Could you check a few things on this model? Use its own coordinates, in mm. A direction names the side the tool comes from. Give positions to 0.01 mm unless a question says otherwise; leave off trailing zeros. Write each loop counter-clockwise with the first axis right and the second up, starting at its lowest first coordinate (ties: lowest second). Pieces come first, ordered by that corner, then holes. Notation, with made-up numbers: M -2,-12 L 45,-12 A22 ccw 45,22 Z; hole C 56.5,81 d1. An arc over 180 degrees is marked long. One line per item, written item: value.
```python
from build123d import *

# Parameters (mm, degrees)
CYLINDER040_R     = 2.5
CYLINDER040_DEPTH = 20
CYLINDER039_R     = 2.5
CYLINDER039_DEPTH = 20
BOX012_W          = 10
BOX012_H          = 12
BOX012_DEPTH      = 120
BOX013_W          = 20
BOX013_H          = 40
BOX013_DEPTH      = 120


with BuildPart() as cilindro027:
    # Cylinder040 → Cylinder040 (new body)
    with BuildSketch(Plane(origin=(-10, 59, 115), x_dir=(0, 0, -1), z_dir=(1, 0, 0))):
        Circle(CYLINDER040_R)
    extrude(amount=CYLINDER040_DEPTH)


with BuildPart() as obj1:
    # Cylinder039 → Cylinder039 (new body)
    with BuildSketch(Plane(origin=(-10, 59, 5), x_dir=(0, 0, -1), z_dir=(1, 0, 0))):
        Circle(CYLINDER039_R)
    extrude(amount=CYLINDER039_DEPTH)

    # Fusion021: union Cilindro027
    add(cilindro027.part)


with BuildPart() as obj1_1:
    # Fusion021 placement: moved
    add(obj1.part.moved(Location((0, -60, 0))))


with BuildPart() as cubo012:
    # Box012 → Box012 (new body)
    with BuildSketch(Plane(origin=(-5, -72, 0), x_dir=(1, 0, 0), z_dir=(0, 0, 1))):
        with Locations((5, 6)):
            Rectangle(BOX012_W, BOX012_H)
    extrude(amount=BOX012_DEPTH)


with BuildPart() as cut037:
    # Box013 → Box013 (new body)
    with BuildSketch(Plane(origin=(-10, -100, 0), x_dir=(1, 0, 0), z_dir=(0, 0, 1))):
        with Locations((10, 20)):
            Rectangle(BOX013_W, BOX013_H)
    extrude(amount=BOX013_DEPTH)

    # Cut036: cut Cubo012
    add(cubo012.part, mode=Mode.SUBTRACT)


with BuildPart() as cut037_1:
    # Cut036 placement: moved
    add(cut037.part.moved(Location((0, 64, 0))))

    # Cut037: cut obj1
    add(obj1_1.part, mode=Mode.SUBTRACT)


solid = cut037_1.part
```
1) If we section it at C-C, the plane z = 101: Write out the boundary of the cut face in (x, y).
Outcome:
outline: M -10,-36 L 10,-36 L 10,4 L 5,4 L 5,-8 L -5,-8 L -5,4 L -10,4 Z
2) Please list where these lines run through material, in increasing order: L1, parallel to Z at x = 8.55, y = -1; L2, parallel to Y at x = 7.45, z = 115; L3, parallel to X at y = -4, z = 80. Write a range as from..to.
Outcome:
L1: z = 0..2.5, 7.5..112.5, 117.5..120
L2: y = -36..-3.5, 1.5..4
L3: x = -10..-5, 5..10
3) If we section it at D-D, the plane x = -3: Write out the boundary of the cut face in (y, z).
Outcome:
outline: M -36,0 L -8,0 L -8,120 L -36,120 Z
4) On a 3-axis mill with a long thin cutter (end or side, diameter ignored), from which of +Z, -Z, +X, -X, +Y, -Y can I reach the whole of each face in a straight line? I mean faces 1 (the face through (-7.535, -0.249, 2.615)), 2 (the face through (-5, -2, 59)). Say none if no direction works.
Outcome:
face 1: +X, -X
face 2: +Z, -Z, +Y
5) If we section it at A-A, the plane z = 115: Write out the boundary of the cut face in (x, y).
Outcome:
outline: M -10,-36 L 10,-36 L 10,-3.5 L 5,-3.5 L 5,-8 L -5,-8 L -5,-3.5 L -10,-3.5 Z; M -10,1.5 L -5,1.5 L -5,4 L -10,4 Z; M 5,1.5 L 10,1.5 L 10,4 L 5,4 Z
6) We'd pull the mould along Z, two halves only. Please class faces 3 (the face through (-7.535, -0.249, 112.615)), 4 (the face through (0, -20, 120)), 5 (the face through (7, 4, 59)): pulls with the +Z half, pulls with the -Z half, needs draft (parallel to the pull), parting line crosses it, or undercut.
Outcome:
face 3: undercut
face 4: pulls with the +Z half
face 5: needs draft
7) I'm going to push flat-ended pins straight in: pin 1 (1.5 mm diameter, centred on x = -1, z = 101.5, fed in from +Y); pin 2 (4.5 mm diameter, centred on y = -1, z = 5, fed in from -X). Where does each tip first touch, or does it pass through?
Outcome:
pin 1: stops at y = -8
pin 2: passes through
8) If we section it at B-B, the plane y = -1: Write out the boundary of the cut face in (x, z), then the cut area to 3 significant figures.
Outcome:
outline: M -10,0 L -5,0 L -5,2.5 L -10,2.5 Z; M -10,7.5 L -5,7.5 L -5,112.5 L -10,112.5 Z; M -10,117.5 L -5,117.5 L -5,120 L -10,120 Z; M 5,0 L 10,0 L 10,2.5 L 5,2.5 Z; M 5,7.5 L 10,7.5 L 10,112.5 L 5,112.5 Z; M 5,117.5 L 10,117.5 L 10,120 L 5,120 Z
area: 1,100 mm^2
